```python
from build123d import *

# Parameters (mm, degrees)
F0_W          = 101.6
F0_H          = 50.8
F1_DEPTH      = 3.175
F3_DEPTH      = 0.254
F5_DEPTH      = 25.4
F5_DEPTH_BACK = 25.4
F6_R          = 2.032
F7_DEPTH      = 25.4
F7_DEPTH_BACK = 25.4


with BuildPart() as f1:
    # F0 (on Top) → F1 (new body)
    with BuildSketch(Plane.XY):
        with Locations((50.9793485571, 25.1952067787)):
            Rectangle(F0_W, F0_H)
    extrude(amount=F1_DEPTH)

    # F2 (on face) → F3 (cut)
    with BuildSketch(Plane.XY.offset(3.175)):
        with BuildLine():
            Line((11.6093485571, 35.9902067787), (11.6093485571, 39.1652067787))
            Line((11.6093485571, 39.1652067787), (14.7843485571, 39.1652067787))
            ThreePointArc((14.7843485571, 39.1652067787), (9.3642845268, 41.4102708089), (11.6093485571, 35.9902067787))
        make_face()
        with BuildLine():
            Line((14.7843485571, 39.1652067787), (11.6093485571, 39.1652067787))
            Line((11.6093485571, 39.1652067787), (11.6093485571, 35.9902067787))
            ThreePointArc((11.6093485571, 35.9902067787), (13.8544125874, 36.9201427484), (14.7843485571, 39.1652067787))
        make_face()
        with BuildLine():
            ThreePointArc((14.7843485571, 11.2252067787), (13.8544125874, 13.4702708089), (11.6093485571, 14.4002067787))
            Line((11.6093485571, 14.4002067787), (11.6093485571, 11.2252067787))
            Line((11.6093485571, 11.2252067787), (14.7843485571, 11.2252067787))
        make_face()
        with BuildLine():
            Line((11.6093485571, 11.2252067787), (11.6093485571, 14.4002067787))
            ThreePointArc((11.6093485571, 14.4002067787), (9.3642845268, 8.9801427484), (14.7843485571, 11.2252067787))
            Line((14.7843485571, 11.2252067787), (11.6093485571, 11.2252067787))
        make_face()
        with BuildLine():
            Line((90.3493485571, 11.2252067787), (90.3493485571, 14.4002067787))
            ThreePointArc((90.3493485571, 14.4002067787), (88.1042845268, 13.4702708089), (87.1743485571, 11.2252067787))
            Line((87.1743485571, 11.2252067787), (90.3493485571, 11.2252067787))
        make_face()
        with BuildLine():
            ThreePointArc((93.5243485571, 11.2252067787), (92.5944125874, 13.4702708089), (90.3493485571, 14.4002067787))
            Line((90.3493485571, 14.4002067787), (90.3493485571, 11.2252067787))
            Line((90.3493485571, 11.2252067787), (87.1743485571, 11.2252067787))
            ThreePointArc((87.1743485571, 11.2252067787), (90.3493485571, 8.0502067787), (93.5243485571, 11.2252067787))
        make_face()
        with BuildLine():
            ThreePointArc((93.5243485571, 39.1652067787), (90.3493485571, 42.3402067787), (87.1743485571, 39.1652067787))
            Line((87.1743485571, 39.1652067787), (90.3493485571, 39.1652067787))
            Line((90.3493485571, 39.1652067787), (90.3493485571, 35.9902067787))
            ThreePointArc((90.3493485571, 35.9902067787), (92.5944125874, 36.9201427484), (93.5243485571, 39.1652067787))
        make_face()
        with BuildLine():
            Line((90.3493485571, 39.1652067787), (87.1743485571, 39.1652067787))
            ThreePointArc((87.1743485571, 39.1652067787), (88.1042845268, 36.9201427484), (90.3493485571, 35.9902067787))
            Line((90.3493485571, 35.9902067787), (90.3493485571, 39.1652067787))
        make_face()
        with BuildLine():
            Line((87.1743485571, 39.1652067787), (14.7843485571, 39.1652067787))
            ThreePointArc((14.7843485571, 39.1652067787), (13.8544125874, 36.9201427484), (11.6093485571, 35.9902067787))
            Line((11.6093485571, 35.9902067787), (11.6093485571, 14.4002067787))
            ThreePointArc((11.6093485571, 14.4002067787), (13.8544125874, 13.4702708089), (14.7843485571, 11.2252067787))
            Line((14.7843485571, 11.2252067787), (87.1743485571, 11.2252067787))
            ThreePointArc((87.1743485571, 11.2252067787), (88.1042845268, 13.4702708089), (90.3493485571, 14.4002067787))
            Line((90.3493485571, 14.4002067787), (90.3493485571, 35.9902067787))
            ThreePointArc((90.3493485571, 35.9902067787), (88.1042845268, 36.9201427484), (87.1743485571, 39.1652067787))
        make_face()
    extrude(amount=-F3_DEPTH, mode=Mode.SUBTRACT)

    # F4 (on face) → F5 (cut, two sides)
    with BuildSketch(Plane.XY.offset(2.921)) as f5_sk:
        with BuildLine():
            ThreePointArc((15.4193485571, 17.5752067787), (16.1632973329, 15.7791555545), (17.9593485571, 15.0352067787))
            Line((17.9593485571, 15.0352067787), (83.9993485571, 15.0352067787))
            ThreePointArc((83.9993485571, 15.0352067787), (85.7953997813, 15.7791555545), (86.5393485571, 17.5752067787))
            Line((86.5393485571, 17.5752067787), (86.5393485571, 32.8152067787))
            ThreePointArc((86.5393485571, 32.8152067787), (85.7953997813, 34.6112580029), (83.9993485571, 35.3552067787))
            Line((83.9993485571, 35.3552067787), (17.9593485571, 35.3552067787))
            ThreePointArc((17.9593485571, 35.3552067787), (16.1632973329, 34.6112580029), (15.4193485571, 32.8152067787))
            Line((15.4193485571, 32.8152067787), (15.4193485571, 17.5752067787))
        make_face()
    extrude(amount=-F5_DEPTH, mode=Mode.SUBTRACT)
    extrude(f5_sk.sketch, amount=F5_DEPTH_BACK, mode=Mode.SUBTRACT)

    # F6 (on face) → F7 (cut, two sides)
    with BuildSketch(Plane.XY.offset(3.175)) as f7_sk:
        with Locations((6.5293485571, 44.2452067787)):
            Circle(F6_R)
        with Locations((95.4293485571, 44.2452067787)):
            Circle(F6_R)
        with Locations((95.4293485571, 6.1452067787)):
            Circle(F6_R)
        with Locations((6.35, 6.35)):
            Circle(F6_R)
    extrude(amount=-F7_DEPTH, mode=Mode.SUBTRACT)
    extrude(f7_sk.sketch, amount=F7_DEPTH_BACK, mode=Mode.SUBTRACT)


solid = f1.part
```
Can you work these out from the model? Positions are in its coordinate system, mm. A direction names the side the tool comes from. Coordinates: 2 decimals unless noted, no trailing zeros. Order: outer loops, then holes, each group sorted by start corner. A loop starts at its lowest first (then second) coordinate and runs counter-clockwise, first axis right, second up.
1. If we section it at B-B (x = 50.5): Please give me the cut outline in (y, z) (3 decimals).
2. If we section it at D-D (z = 1.85): Please give me the cut outline in (x, y).
3. I'm going to push flat-ended pins straight in: pin 1 (6.5 mm diameter, centred on x = 6.53, y = 44.25, fed in from +Z) (3 decimals); pin 2 (2.5 mm diameter, centred on x = 6.35, y = 6.35, fed in from +Z); pin 3 (8 mm diameter, centred on x = 59.5, y = 34, fed in from +Z). Where does each tip first touch, or does it pass through?
4. If we section it at A-A (y = 21): Please give me the cut outline in (x, z) (3 decimals), then the cut area to 3 significant figures.
5. I need wall thicknesses on line 1 (Y direction, x = 44, z = 0.5); line 2 (X direction, y = 18, z = 1.05); line 3 (X direction, y = 8, z = 2.25). Which ranges of each line are inside material? Lowest first, please.
6. If we section it at C-C (x = 6.35): Please give me the cut outline in (y, z) (3 decimals).
7. For faces 4 (the face through (51, 15.035, 1)), 5 (the face through (50, 50.595, 2)), which set-ups out of +Z, -Z, +X, -X, +Y, -Y let a thin tool reach every point of the face, with its end or its side?
8. Thinking about a two-plate mould opening in X: for faces 1 (the face through (0.179, 25, 2)), 2 (the face through (85.815, 34.591, 1.481)), 3 (the face through (50, -0.205, 2)), which applies, +X half, -X half, draft (parallel to the pull), parting line (faces both ways), or undercut?
Entries:
1. outline: (-0.205, 0) - (15.035, 0) - (15.035, 2.921) - (11.225, 2.921) - (11.225, 3.175) - (-0.205, 3.175) - close; (35.355, 0) - (50.595, 0) - (50.595, 3.175) - (39.165, 3.175) - (39.165, 2.921) - (35.355, 2.921) - close
2. outline: (0.18, -0.2) - (101.78, -0.2) - (101.78, 50.6) - (0.18, 50.6) - close; hole circle Ø4.06 at (6.35, 6.35); hole circle Ø4.06 at (6.53, 44.25); hole (15.42, 17.58) arc R2.54 ccw to (17.96, 15.04) - (84, 15.04) arc R2.54 ccw to (86.54, 17.58) - (86.54, 32.82) arc R2.54 ccw to (84, 35.36) - (17.96, 35.36) arc R2.54 ccw to (15.42, 32.82) - close; hole circle Ø4.06 at (95.43, 6.15); hole circle Ø4.06 at (95.43, 44.25)
3. pin 1: stops at z = 3.175
3. pin 2: passes through
3. pin 3: stops at z = 2.92
4. outline: (0.179, 0) - (15.419, 0) - (15.419, 2.921) - (11.609, 2.921) - (11.609, 3.175) - (0.179, 3.175) - close; (86.539, 0) - (101.779, 0) - (101.779, 3.175) - (90.349, 3.175) - (90.349, 2.921) - (86.539, 2.921) - close
4. area: 94.8 mm2
5. line 1: y = -0.2 to 15.04, 35.36 to 50.6
5. line 2: x = 0.18 to 15.42, 86.54 to 101.78
5. line 3: x = 0.18 to 5.16, 7.54 to 94.6, 96.26 to 101.78
6. outline: (-0.205, 0) - (4.318, 0) - (4.318, 3.175) - (-0.205, 3.175) - close; (8.382, 0) - (42.221, 0) - (42.221, 3.175) - (8.382, 3.175) - close; (46.269, 0) - (50.595, 0) - (50.595, 3.175) - (46.269, 3.175) - close
7. face 4: +Z, -Z
7. face 5: +Z, -Z, +X, -X, +Y
8. face 1: -X half
8. face 2: undercut
8. face 3: draft
